from build123d import *

# Parameters (mm, degrees)
EXTRUDE_1_DEPTH     = 205
SKETCH_2_R          = 1
CUT_EXTRUDE_1_DEPTH = 10
CHAMFER_1_SIZE      = 0.5
SKETCH_3_R          = 2.383304988
CUT_EXTRUDE_2_DEPTH = 1


with BuildPart() as part:
    # 草图1 → 凸台-拉伸1 (new body)
    with BuildSketch(Plane(origin=(0, 0, 0), x_dir=(1, 0, 0), z_dir=(0, 1, 0))):
        Polygon((-3.5, 0.4), (-3.5, -2.4), (3.5, -2.4), (3.5, 0.4), (2.5, 0.4), (2.5, 1.4), (3.5, 1.4), (3.5, 2.4), (-3.5, 2.4), (-3.5, 1.4), (-2.5, 1.4), (-2.5, 0.4), align=None)
    extrude(amount=EXTRUDE_1_DEPTH)

    # 草图2 → 切除-拉伸1 (cut)
    with BuildSketch(Plane(origin=(0, 0, -2.4), x_dir=(-1, 0, 0), z_dir=(0, 0, -1))):
        with Locations((0, 5)):
            Circle(SKETCH_2_R)
        with Locations((0, 20)):
            Circle(SKETCH_2_R)
        with Locations((0, 35)):
            Circle(SKETCH_2_R)
        with Locations((0, 50)):
            Circle(SKETCH_2_R)
        with Locations((0, 65)):
            Circle(SKETCH_2_R)
        with Locations((0, 80)):
            Circle(SKETCH_2_R)
        with Locations((0, 95)):
            Circle(SKETCH_2_R)
        with Locations((0, 110)):
            Circle(SKETCH_2_R)
        with Locations((0, 125)):
            Circle(SKETCH_2_R)
        with Locations((0, 140)):
            Circle(SKETCH_2_R)
        with Locations((0, 155)):
            Circle(SKETCH_2_R)
        with Locations((0, 170)):
            Circle(SKETCH_2_R)
        with Locations((0, 185)):
            Circle(SKETCH_2_R)
        with Locations((0, 200)):
            Circle(SKETCH_2_R)
    extrude(amount=-CUT_EXTRUDE_1_DEPTH, mode=Mode.SUBTRACT)

    # 倒角1
    chamfer_1_edges = [part.edges().sort_by_distance(p)[0] for p in [
        (-3.5, 102.5, -2.4),
        (3.5, 102.5, -2.4),
        (3.5, 102.5, 2.4),
        (-3.5, 102.5, 2.4),
    ]]
    chamfer(chamfer_1_edges, length=CHAMFER_1_SIZE)

    # 草图3 → 切除-拉伸2 (cut)
    with BuildSketch(Plane(origin=(0, 0, -2.4), x_dir=(-1, 0, 0), z_dir=(0, 0, -1))):
        with Locations((0, 5)):
            Circle(SKETCH_3_R)
        with Locations((0, 20)):
            Circle(SKETCH_3_R)
        with Locations((0, 35)):
            Circle(SKETCH_3_R)
        with Locations((0, 50)):
            Circle(SKETCH_3_R)
        with Locations((0, 65)):
            Circle(SKETCH_3_R)
        with Locations((0, 80)):
            Circle(SKETCH_3_R)
        with Locations((0, 95)):
            Circle(SKETCH_3_R)
        with Locations((0, 110)):
            Circle(SKETCH_3_R)
        with Locations((0, 125)):
            Circle(SKETCH_3_R)
        with Locations((0, 140)):
            Circle(SKETCH_3_R)
        with Locations((0, 155)):
            Circle(SKETCH_3_R)
        with Locations((0, 170)):
            Circle(SKETCH_3_R)
        with Locations((0, 185)):
            Circle(SKETCH_3_R)
        with Locations((0, 200)):
            Circle(SKETCH_3_R)
    extrude(amount=-CUT_EXTRUDE_2_DEPTH, mode=Mode.SUBTRACT)


solid = part.part
Read the model definition and answer for the solid it produces. Units are mm, in the model's axes. A direction names the side the tool comes from. Coordinates: 2 decimals unless noted, no trailing zeros. Answer in a Markdown table with one row per item.
Q1. Straight lines are drawn through the part: line 1 along X through (y, z) = (140, 0.45); line 2 along Z through (x, y) = (0, 93); line 3 along Z through (x, y) = (3.25, 88.5). For each, find the intervals that lie inside material, in ascending order. Write a range as [from, to].
Here are the results:
| item | result |
|---|---|
| line 1 | x = [-3.5, -1], [1, 3.5] |
| line 2 | z = [-1.4, 2.4] |
| line 3 | z = [-2.15, -1.4], [-0.4, 2.15] |
Q2. Given P1, Ø1.4, axis at x = 0.5, y = 6, coming from the -Z side, flat-ended and moving along its own axis, determine where the tip first touches the part or whether it passes through.
Here are the results:
| item | result |
|---|---|
| P1 | stops at z = -1.4 |
Q3. The mould has two halves that part along X. Classify faces 3 (the flat face through (0, 101, 2.4)), 4 (the cylindrical face through (0.517, 107.673, -1.907)): pulls with the +X half, pulls with the -X half, needs draft (parallel to the pull), parting line crosses it, or undercut.
Here are the results:
| item | result |
|---|---|
| face 3 | needs draft |
| face 4 | undercut |
Q4. Find section A-A on z = 0.4. Count the separate pieces of the cut face and the enclosed holes in it, plus the area to 3 significant figures.
Here are the results:
| item | result |
|---|---|
| separate pieces | 1 |
| enclosed holes | 14 |
| area | 1,390 mm^2 |
Q5. For faces 1 (the flat face through (0, 101, -2.4)), 2 (the cylindrical face through (1.89, 33.55, -1.91)), determine the directions among +Z, -Z, +X, -X, +Y, -Y from which every point of the face is accessible in a straight line to the end or side of a thin tool.
Here are the results:
| item | result |
|---|---|
| face 1 | -Z, +X, -X, +Y, -Y |
| face 2 | -Z |
